from build123d import *

# Parameters (mm, degrees)
SKETCH_W  = 235
SKETCH_H  = 235
PAD_DEPTH = 50


with BuildPart() as part:
    # Sketch → Pad (new body)
    with BuildSketch(Plane.XY):
        Rectangle(SKETCH_W, SKETCH_H)
        with BuildLine():
            Line((62.5, -62.5), (62.5, -35.355339))
            ThreePointArc((62.5, -35.355339), (105.17767, -17.677671), (62.500003, 3e-06))
            ThreePointArc((62.5, 35.355339), (19.82233, 17.677668), (62.500003, 3e-06))
            Line((62.5, 35.355339), (62.5, 62.5))
            Line((62.5, 62.5), (35.355339, 62.5))
            ThreePointArc((35.355339, 62.5), (17.67769, 105.17767), (-2.9e-05, 62.500029))
            ThreePointArc((-35.355339, 62.5), (-17.677649, 19.82233), (-2.9e-05, 62.500029))
            Line((-35.355339, 62.5), (-62.5, 62.5))
            Line((-62.5, 62.5), (-62.5, 35.35541))
            ThreePointArc((-62.5, 35.35541), (-105.177634, 17.67768), (-62.499965, 3.5e-05))
            ThreePointArc((-62.5, -35.355269), (-19.822295, -17.677659), (-62.499965, 3.5e-05))
            Line((-62.5, -35.355269), (-62.5, -62.5))
            Line((-62.5, -62.5), (-35.355339, -62.5))
            ThreePointArc((-35.355339, -62.5), (-17.677671, -105.17767), (3e-06, -62.500003))
            ThreePointArc((35.355339, -62.5), (17.677668, -19.82233), (3e-06, -62.500003))
            Line((35.355339, -62.5), (62.5, -62.5))
        make_face(mode=Mode.SUBTRACT)
    extrude(amount=PAD_DEPTH)


solid = part.part
Here's how the part is built. I have some questions about the finished solid (model axes, mm). A direction names the side the tool comes from. Coordinates: 2 decimals unless noted, no trailing zeros. Write each loop counter-clockwise with the first axis right and the second up, starting at its lowest first coordinate (ties: lowest second). Pieces come first, ordered by that corner, then holes. Notation, with made-up numbers: (54.25, 58) - (98.25, 58) arc R29 ccw to (98.25, 89) - close; hole circle Ø4 at (-15, 68.5). An arc over 180 degrees is marked (long way). Use one line per item in the form item = value.
1) Suppose I cut it at D-D, the plane x = 83.5. Write out the boundary of the cut face in (y, z).
Solved:
outline = (-117.5, 0) - (-42.46, 0) - (-42.46, 50) - (-117.5, 50) - close; (7.1, 0) - (117.5, 0) - (117.5, 50) - (7.1, 50) - close
2) I need wall thicknesses on line 1 (Y direction, x = -25, z = 26); line 2 (Y direction, x = 1, z = 27); line 3 (X direction, y = -17, z = 38.5). Which ranges of each line are inside material? Lowest first, please.
Solved:
line_1 = -117.5 to -104.08, -32.91 to -2.44, 20.92 to 117.5
line_2 = -117.5 to -96.8, -63.56 to -26.2, 28.2 to 61.44, 98.8 to 117.5
line_3 = -117.5 to -19.83, 105.17 to 117.5
3) Suppose I cut it at C-C, the plane z = 35.5. Write out the boundary of the cut face in (x, y), plus the area to 3 significant figures.
Solved:
outline = (-117.5, -117.5) - (117.5, -117.5) - (117.5, 117.5) - (-117.5, 117.5) - close; hole (-62.5, -62.5) - (-35.36, -62.5) arc R25 ccw (long way) to (0, -62.5) arc R25 cw (long way) to (35.36, -62.5) - (62.5, -62.5) - (62.5, -35.36) arc R25 ccw (long way) to (62.5, 0) arc R25 cw (long way) to (62.5, 35.36) - (62.5, 62.5) - (35.36, 62.5) arc R25 ccw (long way) to (0, 62.5) arc R25 cw (long way) to (-35.36, 62.5) - (-62.5, 62.5) - (-62.5, 35.36) arc R25 ccw (long way) to (-62.5, 0) arc R25 cw (long way) to (-62.5, -35.36) - close
area = 39,600 mm2
4) On a 3-axis mill with a long thin cutter (end or side, diameter ignored), from which of +Z, -Z, +X, -X, +Y, -Y can I reach the whole of each face in a straight line? I mean faces 4 (the flat face through (-117.5, -2, 25)), 5 (the flat face through (49, -62.5, 25)). Say none if no direction works.
Solved:
face_4 = +Z, -Z, -X, +Y, -Y
face_5 = +Z, -Z
5) Suppose I cut it at B-B, the plane y = -54.5. Write out the boundary of the cut face in (x, z).
Solved:
outline = (-117.5, 0) - (-62.5, 0) - (-62.5, 50) - (-117.5, 50) - close; (-5.37, 0) - (40.73, 0) - (40.73, 50) - (-5.37, 50) - close; (62.5, 0) - (117.5, 0) - (117.5, 50) - (62.5, 50) - close
6) Thinking about a two-plate mould opening in Y: for faces 1 (the flat face through (62.5, -49, 25)), 2 (the flat face through (117.5, -2, 25)), 3 (the flat face through (-2, 117.5, 25)), which applies, released by +Y, released by -Y, zero draft, split by the parting line, or undercut?
Solved:
face_1 = undercut
face_2 = zero draft
face_3 = released by +Y
7) Suppose I cut it at A-A, the plane x = -48. Write out the boundary of the cut face in (y, z).
Solved:
outline = (-117.5, 0) - (-62.5, 0) - (-62.5, 50) - (-117.5, 50) - close; (-42.47, 0) - (7.12, 0) - (7.12, 50) - (-42.47, 50) - close; (62.5, 0) - (117.5, 0) - (117.5, 50) - (62.5, 50) - close
